```python
from build123d import *

# Parameters (mm, degrees)
F0_W     = 106.68
F0_H     = 25.4
F2_R     = 6.223
F3_DEPTH = 12.7
F4_R     = 6.35
F5_DEPTH = 12.7


with BuildPart() as f1:
    # F0 (on Top) → F1 (revolve)
    with BuildSketch(Plane.XY):
        with Locations((-0.314683, -23.51072)):
            Rectangle(F0_W, F0_H)
    revolve(axis=Axis((-0.314683, -10.81072, 0), (1, 0, 0)))

    # F2 (on face) → F3 (join)
    with BuildSketch(Plane(origin=(-53.654683, 0, 0), x_dir=(0, -1, 0), z_dir=(-1, 0, 0))):
        with Locations((10.81072, 0)):
            Circle(F2_R)
    extrude(amount=F3_DEPTH)

    # F4 (on face) → F5 (join)
    with BuildSketch(Plane.YZ.offset(53.025317)):
        with Locations((-10.81072, 0)):
            Circle(F4_R)
    extrude(amount=F5_DEPTH)


solid = f1.part
```
The model under review builds one solid part; all positions refer to its coordinate system, in mm. A direction names the side the tool comes from. Give positions to 0.01 mm unless a question says otherwise; leave off trailing zeros. Write each loop counter-clockwise with the first axis right and the second up, starting at its lowest first coordinate (ties: lowest second). Pieces come first, ordered by that corner, then holes. Notation, with made-up numbers: (54, -30.75) -> (71, -30.75) arc R18 ccw to (71, 1.25) -> close; hole circle Ø11 at (-4, -21.5). An arc over 180 degrees is marked (long way). Answer in a Markdown table with one row per item.
1) Tool access review of faces 1 (the cylindrical face through (-59.92, -16.56, -2.38)), 2 (the flat face through (65.725, -11, 0)), 3 (the flat face through (53.025, -16, 5)): name each direction out of +Z, -Z, +X, -X, +Y, -Y from which nothing blocks a thin tool from reaching the whole face with its end or side.
Worked answers:
| item | result |
|---|---|
| face 1 | -X |
| face 2 | +Z, -Z, +X, +Y, -Y |
| face 3 | +X |
2) Add section C-C on y = -31.5. State the section outline as (x, z) points, plus the area to 3 significant figures.
Worked answers:
| item | result |
|---|---|
| outline | (-53.65, -14.73) -> (53.03, -14.73) -> (53.03, 14.73) -> (-53.65, 14.73) -> close |
| area | 3,140 mm² |
3) Add section B-B on x = 43. State the section outline as (y, z) points, plus the area to 3 significant figures.
Worked answers:
| item | result |
|---|---|
| outline | circle Ø50.8 at (-10.81, 0) |
| area | 2,030 mm² |
4) Clearance check with flat-ended pins moving along their axes: P1, Ø5, axis at x = 37.5, y = -1, coming from the -Z side; P2, Ø4, axis at x = -45.5, z = -12, coming from the -Y side; P3, Ø1, axis at y = -7, z = -14, coming from the -X side. State where each tip first meets the part, or that it passes through.
Worked answers:
| item | result |
|---|---|
| P1 | z = -24.33 |
| P2 | y = -34.16 |
| P3 | x = -53.65 |
5) For L1, parallel to X at y = -19, z = -13; L2, parallel to Z at x = -16.5, y = -11.5; L3, parallel to Z at x = -46.5, y = -33.5, list the stretches that pass through material, from the lowest coordinate up. Write a range as [from, to].
Worked answers:
| item | result |
|---|---|
| L1 | [-53.65, 53.03] |
| L2 | [-25.39, 25.39] |
| L3 | [-11.42, 11.42] |
6) Add section A-A on z = 0. State the section outline as (x, y) points.
Worked answers:
| item | result |
|---|---|
| outline | (-66.35, -17.03) -> (-53.65, -17.03) -> (-53.65, -36.21) -> (53.03, -36.21) -> (53.03, -17.16) -> (65.73, -17.16) -> (65.73, -4.46) -> (53.03, -4.46) -> (53.03, 14.59) -> (-53.65, 14.59) -> (-53.65, -4.59) -> (-66.35, -4.59) -> close |
7) Add section D-D on z = -12. State the section outline as (x, y) points, plus the area to 3 significant figures.
Worked answers:
| item | result |
|---|---|
| outline | (-53.65, -33.2) -> (53.03, -33.2) -> (53.03, 11.58) -> (-53.65, 11.58) -> close |
| area | 4,780 mm² |
